Design review of the part built by this model. Coordinates are the model's own, in mm. A direction names the side the tool comes from. Coordinates: 2 decimals unless noted, no trailing zeros. Write each loop counter-clockwise with the first axis right and the second up, starting at its lowest first coordinate (ties: lowest second). Pieces come first, ordered by that corner, then holes. Notation, with made-up numbers: (45, 41) - (51, 41) arc R20 cw to (51, 74) - close; hole circle Ø7 at (-28.75, 83). An arc over 180 degrees is marked (long way). Answer as CSV lines item,"result". Start each with the question number.
Q1. Machinability: for faces 1 (the face through (9.75, 10.54, 11.5)), 2 (the face through (10, -7, -6)), 3 (the face through (0.25, 10.54, -11.5)), which of the approach directions +Z, -Z, +X, -X, +Y, -Y give a long, thin tool a straight path to every point of the face, cutting with its end or side? Answer none if there is none.
Q2. Clearance check with flat-ended pins moving along their axes: pin 1 (1 mm diameter, centred on y = 4, z = 7, fed in from -X); pin 2 (1.5 mm diameter, centred on x = 3.5, y = -8.5, fed in from +Z); pin 3 (1 mm diameter, centred on x = 1, y = -8.5, fed in from -Z). State where each tip first meets the part, or that it passes through.
Q3. For line 1 along Y through (x, z) = (6.5, 0); line 2 along Y through (x, z) = (0.3, 0) (3 decimals); line 3 along Y through (x, z) = (9.95, 0) (3 decimals), list the stretches that pass through material, from the lowest coordinate up. Write a range as [from, to].
Q4. We need section C-C (x = 8.75). Write out the cut boundary in (y, z), plus the area to 3 significant figures.
from build123d import *

# Parameters (mm, degrees)
SKETCH1_R           = 17.5
SKETCH1_R_2         = 8.5
BOSS_EXTRUDE1_DEPTH = 10
CHAMFER1_SIZE       = 0.5
SKETCH2_R           = 15.6
SKETCH2_R_2         = 10.225
CUT_EXTRUDE1_DEPTH  = 0.5
SKETCH3_R           = 15.6
SKETCH3_R_2         = 10.225
CUT_EXTRUDE2_DEPTH  = 0.5


with BuildPart() as part:
    # Sketch1 → Boss-Extrude1 (new body)
    with BuildSketch(Plane(origin=(0, 0, 0), x_dir=(0, 0, -1), z_dir=(1, 0, 0))):
        Circle(SKETCH1_R)
        Circle(SKETCH1_R_2, mode=Mode.SUBTRACT)
    extrude(amount=BOSS_EXTRUDE1_DEPTH)

    # Chamfer1
    chamfer1_edges = [part.edges().sort_by_distance(p)[0] for p in [
        (0, 0, 17.5),
        (10, 0, 17.5),
        (0, 0, 8.5),
        (10, 0, 8.5),
    ]]
    chamfer(chamfer1_edges, length=CHAMFER1_SIZE)

    # Sketch2 → Cut-Extrude1 (cut)
    with BuildSketch(Plane(origin=(10, 0, 0), x_dir=(0, 0, -1), z_dir=(1, 0, 0))):
        Circle(SKETCH2_R)
        Circle(SKETCH2_R_2, mode=Mode.SUBTRACT)
    extrude(amount=-CUT_EXTRUDE1_DEPTH, mode=Mode.SUBTRACT)

    # Sketch3 → Cut-Extrude2 (cut)
    with BuildSketch(Plane.ZY):
        Circle(SKETCH3_R)
        Circle(SKETCH3_R_2, mode=Mode.SUBTRACT)
    extrude(amount=-CUT_EXTRUDE2_DEPTH, mode=Mode.SUBTRACT)


solid = part.part
Results list:
1,face 1,"+X"
1,face 2,"+Z, -Z, +X, +Y, -Y"
1,face 3,"-X"
2,pin 1,"stops at x = 0.44"
2,pin 2,"stops at z = 15.69"
2,pin 3,"stops at z = -15.56"
3,line 1,"y = [-17.5, -8.5], [8.5, 17.5]"
3,line 2,"y = [-17.3, -15.6], [-10.225, -8.7], [8.7, 10.225], [15.6, 17.3]"
3,line 3,"y = [-17.05, -15.6], [-10.225, -8.95], [8.95, 10.225], [15.6, 17.05]"
4,outline,"circle Ø35 at (0, 0); hole circle Ø17 at (0, 0)"
4,area,"735 mm2"
